```python
from build123d import *

# Parameters (mm, degrees)
SKETCH2_R          = 1.65
CUT_EXTRUDE1_DEPTH = 10
SKETCH3_R          = 3
CUT_EXTRUDE2_DEPTH = 4


with BuildPart() as part:
    # Sketch1 → Revolve1 (revolve)
    with BuildSketch(Plane.XY, mode=Mode.PRIVATE) as revolve1_sk:
        Polygon((0, -7), (6.5, -7), (5, 0), (0, 0), align=None)
    revolve(revolve1_sk.sketch.rotate(Axis((0, 0, 0), (0, -1, 0)), 180), axis=Axis((0, 0, 0), (0, -1, 0)))

    # Sketch2 → Cut-Extrude1 (cut)
    with BuildSketch(Plane(origin=(0, 0, 0), x_dir=(1, 0, 0), z_dir=(0, 1, 0))):
        with Locations(Location((0, 0, 0), (0, 0, 180))):
            Circle(SKETCH2_R)
    extrude(amount=-CUT_EXTRUDE1_DEPTH, mode=Mode.SUBTRACT)

    # Sketch3 → Cut-Extrude2 (cut)
    with BuildSketch(Plane(origin=(0, 0, 0), x_dir=(1, 0, 0), z_dir=(0, 1, 0))):
        with Locations(Location((0, 0, 0), (0, 0, 180))):
            Circle(SKETCH3_R)
    extrude(amount=-CUT_EXTRUDE2_DEPTH, mode=Mode.SUBTRACT)


solid = part.part
```
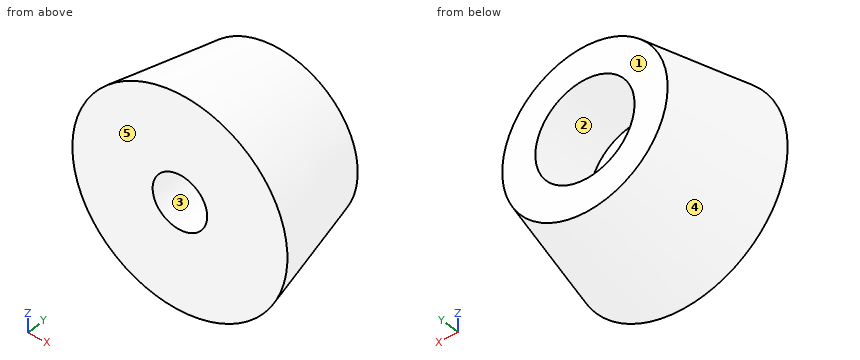
Source: CAD feature listing. Evaluate the final solid. Frame: model axes, mm. Face numbers are marked on the shaded views. A direction names the side the tool comes from. Round coordinates to 2 decimals unless told otherwise and drop trailing zeros. Write each loop counter-clockwise with the first axis right and the second up, starting at its lowest first coordinate (ties: lowest second). Pieces come first, ordered by that corner, then holes. Notation, with made-up numbers: M -1,3.25 L 30,3.25 A16 ccw 30,17.25 Z; hole C 53.5,67 d8. An arc over 180 degrees is marked long. Use CSV: the item, a comma, the result in double quotes. Start each with the question number.
Q1. Cut plane C-C on y = -2.75. Output: boundary loops of the cut face in (x, z), plus the area to 3 significant figures.
Q2. Pull-direction query (X, two-part tool) for the marked faces 3, 4 and 5; classes: +X half, -X half, draft (parallel to the pull), parting line (faces both ways), or undercut.
Q3. Cut plane D-D on y = -2. Output: boundary loops of the cut face in (x, z), plus the area to 3 significant figures.
Q4. First-contact query: P1, Ø3, axis at x = -5, y = -5, coming from the -Z side; P2, Ø4, axis at y = -4, z = 3, coming from the -X side; P3, Ø1.5, axis at x = -3, y = -3.5, coming from the +Z side. Flat tips, straight axial feed; report the tip coordinate or a pass-through.
Q5. Cut plane A-A on z = 0. Output: boundary loops of the cut face in (x, y), plus the area to 3 significant figures.
Q6. Access query for the marked faces 1 and 2. Directions: +Z, -Z, +X, -X, +Y, -Y. A direction counts if a zero-diameter tool reaches every point of the face in a straight line with its end or side. Return the directions, or none.
Q7. Line query: line 1 (Y direction, x = -0.5, z = -2.25); line 2 (Z direction, x = 0.25, y = -2.25); line 3 (Z direction, x = 0, y = -1.9). Output: solid intervals per line, ascending. Write a range as from..to.
Q8. Cut plane B-B on x = 0. Output: boundary loops of the cut face in (y, z).
Results found:
1,outline,"C 0,0 d11.18; hole C 0,0 d6"
1,area,"69.9 mm^2"
2,face 3,"undercut"
2,face 4,"parting line"
2,face 5,"draft"
3,outline,"C 0,0 d10.86; hole C 0,0 d6"
3,area,"64.3 mm^2"
4,P1,"z = -5.03"
4,P2,"x = -5.95"
4,P3,"z = 5.34"
5,outline,"M -6.5,-7 L -1.65,-7 L -1.65,-4 L -3,-4 L -3,0 L -5,0 Z; M 1.65,-7 L 6.5,-7 L 5,0 L 3,0 L 3,-4 L 1.65,-4 Z"
5,area,"46.6 mm^2"
6,face 1,"+Z, -Z, +X, -X, +Y"
6,face 2,"+Y"
7,line 1,"-7..-4"
7,line 2,"-5.48..-2.99, 2.99..5.48"
7,line 3,"-5.41..-3, 3..5.41"
8,outline,"M -7,-6.5 L 0,-5 L 0,-3 L -4,-3 L -4,-1.65 L -7,-1.65 Z; M -7,1.65 L -4,1.65 L -4,3 L 0,3 L 0,5 L -7,6.5 Z"
